The model under review builds one solid part; all positions refer to its coordinate system, in mm. Round coordinates to 2 decimals unless told otherwise and drop trailing zeros. Order: outer loops, then holes, each group sorted by start corner. A loop starts at its lowest first (then second) coordinate and runs counter-clockwise, first axis right, second up.
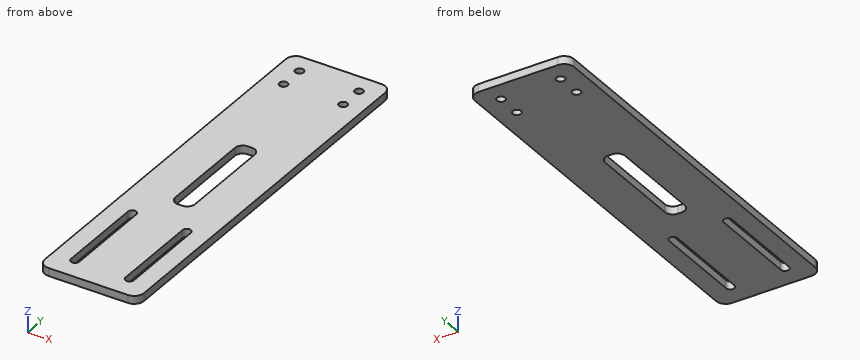
```python
from build123d import *

# Parameters (mm, degrees)
SKETCH1_R          = 4.2
BASE_FLANGE1_DEPTH = 8


# Sheet-metal steps are written as plain solids
with BuildPart() as part:
    # Sketch1 → Base-Flange1 (new body)
    with BuildSketch(Plane.XY):
        with BuildLine():
            Line((-40, 200), (40, 200))
            ThreePointArc((40, 200), (47.071067812, 197.071067812), (50, 190))
            Line((50, 190), (50, -190))
            ThreePointArc((50, -190), (47.071067812, -197.071067812), (40, -200))
            Line((40, -200), (-40, -200))
            ThreePointArc((-40, -200), (-47.071067812, -197.071067812), (-50, -190))
            Line((-50, -190), (-50, 190))
            ThreePointArc((-50, 190), (-47.071067812, 197.071067812), (-40, 200))
        make_face()
        with Locations((30, 180)):
            Circle(SKETCH1_R, mode=Mode.SUBTRACT)
        with Locations((30, 155)):
            Circle(SKETCH1_R, mode=Mode.SUBTRACT)
        with Locations((-30, 180)):
            Circle(SKETCH1_R, mode=Mode.SUBTRACT)
        with Locations((-30, 155)):
            Circle(SKETCH1_R, mode=Mode.SUBTRACT)
        with BuildLine():
            Line((23.3, -87.5), (23.3, -177.5))
            ThreePointArc((23.3, -177.5), (27.5, -181.7), (31.7, -177.5))
            Line((31.7, -177.5), (31.7, -87.5))
            ThreePointArc((31.7, -87.5), (27.5, -83.3), (23.3, -87.5))
        make_face(mode=Mode.SUBTRACT)
        with BuildLine():
            Line((-23.3, -177.5), (-23.3, -87.5))
            ThreePointArc((-23.3, -87.5), (-27.5, -83.3), (-31.7, -87.5))
            Line((-31.7, -87.5), (-31.7, -177.5))
            ThreePointArc((-31.7, -177.5), (-27.5, -181.7), (-23.3, -177.5))
        make_face(mode=Mode.SUBTRACT)
        with BuildLine():
            Line((-2, -55), (2, -55))
            ThreePointArc((2, -55), (7.656854249, -52.656854249), (10, -47))
            Line((10, -47), (10, 47))
            ThreePointArc((10, 47), (7.656854249, 52.656854249), (2, 55))
            Line((2, 55), (-2, 55))
            ThreePointArc((-2, 55), (-7.656854249, 52.656854249), (-10, 47))
            Line((-10, 47), (-10, -47))
            ThreePointArc((-10, -47), (-7.656854249, -52.656854249), (-2, -55))
        make_face(mode=Mode.SUBTRACT)
    extrude(amount=-BASE_FLANGE1_DEPTH)


solid = part.part
```
(1) Consider section A-A (y = 155). Write out the cut boundary in (x, z), and give its area (3 significant figures).
Data:
outline: (-50, -8) - (-34.2, -8) - (-34.2, 0) - (-50, 0) - close; (-25.8, -8) - (25.8, -8) - (25.8, 0) - (-25.8, 0) - close; (34.2, -8) - (50, -8) - (50, 0) - (34.2, 0) - close
area: 666 mm2
(2) Insertion check: pin 1 (4 mm diameter, centred on x = 32, y = -68, fed in from +Z). The pin has a flat end and moves straight along its axis. Give the tip position at first contact, or say it passes through.
Data:
pin 1: stops at z = 0
(3) Consider section B-B (z = -6.5). Write out the cut boundary in (x, y), and give its area (3 significant figures).
Data:
outline: (-50, -190) arc R10 ccw to (-40, -200) - (40, -200) arc R10 ccw to (50, -190) - (50, 190) arc R10 ccw to (40, 200) - (-40, 200) arc R10 ccw to (-50, 190) - close; hole circle Ø8.4 at (-30, 155); hole circle Ø8.4 at (-30, 180); hole (-31.7, -177.5) arc R4.2 ccw to (-23.3, -177.5) - (-23.3, -87.5) arc R4.2 ccw to (-31.7, -87.5) - close; hole (-10, -47) arc R8 ccw to (-2, -55) - (2, -55) arc R8 ccw to (10, -47) - (10, 47) arc R8 ccw to (2, 55) - (-2, 55) arc R8 ccw to (-10, 47) - close; hole (23.3, -177.5) arc R4.2 ccw to (31.7, -177.5) - (31.7, -87.5) arc R4.2 ccw to (23.3, -87.5) - close; hole circle Ø8.4 at (30, 155); hole circle Ø8.4 at (30, 180)
area: 35,900 mm2
(4) Consider section C-C (y = 50.5). Write out the cut boundary in (x, z), and give its area (3 significant figures).
Data:
outline: (-50, -8) - (-9.19, -8) - (-9.19, 0) - (-50, 0) - close; (9.19, -8) - (50, -8) - (50, 0) - (9.19, 0) - close
area: 653 mm2
(5) To check wall thickness, follow probe 1 along X at (y, z) = (-164.5, -3.25); probe 2 along Y at (x, z) = (-1.5, -7.25); probe 3 along Y at (x, z) = (-30, -2.5). State the ranges of each line that lie inside material, in increasing order.
Data:
probe 1: x = -50 to -31.7, -23.3 to 23.3, 31.7 to 50
probe 2: y = -200 to -55, 55 to 200
probe 3: y = -200 to -180.87, -84.13 to 150.8, 159.2 to 175.8, 184.2 to 200
